Geometry check sheet. Reference: drawing and pictorial views, mm from the part's lowest x, y, z. A direction names the side the tool comes from. Coordinates: 2 decimals unless noted, no trailing zeros. Loops run counter-clockwise (first coordinate to the right, second up) from the corner with the lowest first, then second, coordinate; pieces in that order, holes last. Notation, with made-up numbers: M 84.5,-27.75 L 125.5,-27.75 A19 ccw 125.5,-17.75 Z; hole C -4.5,63.5 d7. An arc over 180 degrees is marked long. Write item = value, one per line. Start each with the question number.
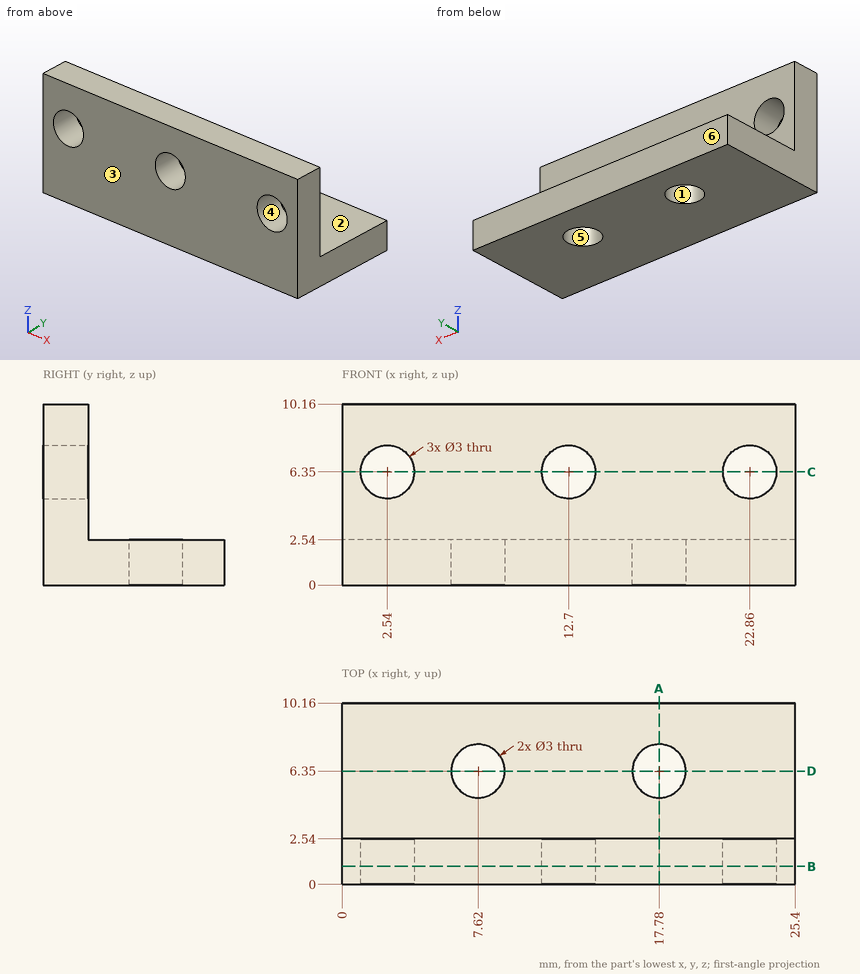
Q1. Sectioned sample at C-C on z = 6.35. Record the cut outline in (x, y).
Q2. Gauge pin test, flat ends, axial feed: pin 1 (6 mm diameter, centred on x = 4, z = 8, fed in from +Y); pin 2 (5 mm diameter, centred on y = 6.5, z = 7, fed in from +X); pin 3 (4 mm diameter, centred on x = 16, y = 5, fed in from +Z). Record the tip position at first contact, or that the pin passes through.
Q3. Sectioned sample at B-B on y = 1. Record the cut outline in (x, z).
Q4. Set-up check for the marked faces 1 and 2: record each of +Z, -Z, +X, -X, +Y, -Y from which the full face is reachable in a straight line by a thin tool's end or side.
Q5. Sectioned sample at D-D on y = 6.35. Record the cut outline in (x, z).
Q6. Sectioned sample at A-A on x = 17.78. Record the cut outline in (y, z), plus the area to 3 significant figures.
Q7. Scan lines: L1, parallel to X at y = 6.25, z = 1.25; L2, parallel to X at y = 1.1, z = 6.35; L3, parallel to Z at x = 2.54, y = 1.2. Record each from-to range of solid material in increasing order. Write a range as [from, to].
Q8. Mould release check, pull along Y, two halves, no side actions. Record for the marked faces 3, 4, 5 and 6: +Y half, -Y half, draft (parallel to the pull), parting line (faces both ways), or undercut.
Solutions:
q1.outline = M 0,0 L 1.04,0 L 1.04,2.54 L 0,2.54 Z; M 4.04,0 L 11.2,0 L 11.2,2.54 L 4.04,2.54 Z; M 14.2,0 L 21.36,0 L 21.36,2.54 L 14.2,2.54 Z; M 24.36,0 L 25.4,0 L 25.4,2.54 L 24.36,2.54 Z
q2.pin_1 = 2.54
q2.pin_2 = through
q2.pin_3 = 2.54
q3.outline = M 0,0 L 25.4,0 L 25.4,10.16 L 0,10.16 Z; hole C 2.54,6.35 d3; hole C 12.7,6.35 d3; hole C 22.86,6.35 d3
q4.face_1 = +Z, -Z
q4.face_2 = +Z, +X, -X, +Y
q5.outline = M 0,0 L 6.12,0 L 6.12,2.54 L 0,2.54 Z; M 9.12,0 L 16.28,0 L 16.28,2.54 L 9.12,2.54 Z; M 19.28,0 L 25.4,0 L 25.4,2.54 L 19.28,2.54 Z
q6.outline = M 0,0 L 4.85,0 L 4.85,2.54 L 2.54,2.54 L 2.54,10.16 L 0,10.16 Z; M 7.85,0 L 10.16,0 L 10.16,2.54 L 7.85,2.54 Z
q6.area = 37.5 mm²
q7.L1 = [0, 6.12], [9.12, 16.28], [19.28, 25.4]
q7.L2 = [0, 1.04], [4.04, 11.2], [14.2, 21.36], [24.36, 25.4]
q7.L3 = [0, 4.85], [7.85, 10.16]
q8.face_3 = -Y half
q8.face_4 = draft
q8.face_5 = undercut
q8.face_6 = +Y half
